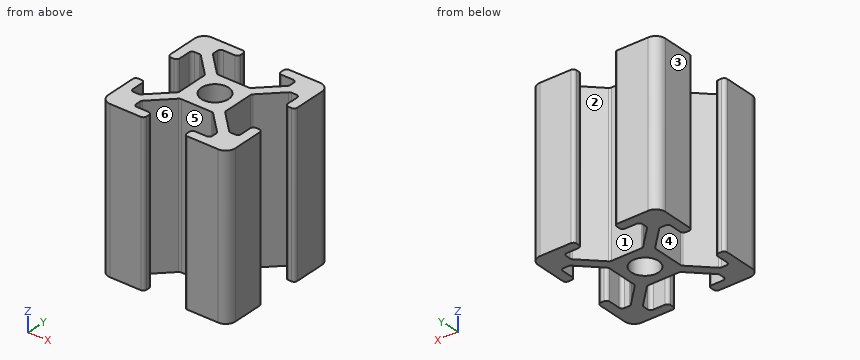
from build123d import *

# Parameters (mm, degrees)
F0_W     = 20
F0_H     = 20
F0_R     = 2.15
F2_DEPTH = 25
F3_DEPTH = 25.001
F4_R     = 1.5
F5_R     = 0.5


with BuildPart() as f2:
    # F0 (on Top) → F2 (new body)
    with BuildSketch(Plane.XY):
        Rectangle(F0_W, F0_H)
        Circle(F0_R, mode=Mode.SUBTRACT)
    extrude(amount=F2_DEPTH)

    # F1 (on face) → F3 (cut, through all)
    with BuildSketch(Plane.XY):
        Polygon((-8.5, 3.18), (-10, 3.18), (-10, -3.18), (-8.5, -3.18), (-8.5, -6), (-7.06066, -6), (-3.65, -2.58934), (-3.65, 2.58934), (-7.06066, 6), (-8.5, 6), align=None)
        Polygon((-3.18, -8.5), (-3.18, -10), (3.18, -10), (3.18, -8.5), (6, -8.5), (6, -7.06066), (2.58934, -3.65), (-2.58934, -3.65), (-6, -7.06066), (-6, -8.5), align=None)
        Polygon((10, -3.18), (10, 3.18), (8.5, 3.18), (8.5, 6), (7.06066, 6), (3.65, 2.58934), (3.65, -2.58934), (7.06066, -6), (8.5, -6), (8.5, -3.18), align=None)
        Polygon((3.18, 10), (-3.18, 10), (-3.18, 8.5), (-6, 8.5), (-6, 7.06066), (-2.58934, 3.65), (2.58934, 3.65), (6, 7.06066), (6, 8.5), (3.18, 8.5), align=None)
    extrude(amount=F3_DEPTH, mode=Mode.SUBTRACT)

    # F4
    f4_edges = [f2.edges().sort_by_distance(p)[0] for p in [
        (10, -10, 12.5),
        (-10, -10, 12.5),
        (10, 10, 12.5),
        (-10, 10, 12.5),
    ]]
    fillet(f4_edges, radius=F4_R)

    # F5
    f5_edges = [f2.edges().sort_by_distance(p)[0] for p in [
        (-3.18, -10, 12.5),
        (-10, 3.18, 12.5),
        (-3.18, 10, 12.5),
        (3.18, -10, 12.5),
        (10, 3.18, 12.5),
        (10, -3.18, 12.5),
        (-10, -3.18, 12.5),
        (3.18, 10, 12.5),
        (-6, -8.5, 12.5),
        (-3.18, -8.5, 12.5),
        (3.18, -8.5, 12.5),
        (-8.5, 3.18, 12.5),
        (-8.5, -3.18, 12.5),
        (8.5, -3.18, 12.5),
        (8.5, 3.18, 12.5),
        (3.18, 8.5, 12.5),
        (6, 8.5, 12.5),
        (8.5, 6, 12.5),
        (7.06066, 6, 12.5),
        (6, 7.06066, 12.5),
        (-2.58934, -3.65, 12.5),
        (2.58934, -3.65, 12.5),
        (3.65, 2.58934, 12.5),
        (3.65, -2.58934, 12.5),
        (-3.65, -2.58934, 12.5),
        (-3.65, 2.58934, 12.5),
        (2.58934, 3.65, 12.5),
        (-2.58934, 3.65, 12.5),
        (-6, 8.5, 12.5),
        (-6, 7.06066, 12.5),
        (-3.18, 8.5, 12.5),
        (8.5, -6, 12.5),
        (7.06066, -6, 12.5),
        (-8.5, -6, 12.5),
        (-7.06066, -6, 12.5),
        (-6, -7.06066, 12.5),
        (6, -7.06066, 12.5),
        (6, -8.5, 12.5),
        (-8.5, 6, 12.5),
        (-7.06066, 6, 12.5),
    ]]
    fillet(f5_edges, radius=F5_R)


solid = f2.part
Can you work these out from the model? Positions are in its coordinate system, mm. Face numbers are marked on the shaded views. A direction names the side the tool comes from. Give positions to 0.01 mm unless a question says otherwise; leave off trailing zeros. Order: outer loops, then holes, each group sorted by start corner. A loop starts at its lowest first (then second) coordinate and runs counter-clockwise, first axis right, second up. Notation, with made-up numbers: M 77.5,56 L 111.5,56 A19 ccw 111.5,81 Z; hole C 13.25,86.5 d10. An arc over 180 degrees is marked long. Use one line per item in the form item = value. Start each with the question number.
Item 1: For the marked faces 4, 5 and 6, which set-ups out of +Z, -Z, +X, -X, +Y, -Y let a thin tool reach every point of the face, with its end or its side?
Item 2: Will these pins go through, and if not, where does the flat tip stop? pin 1 Ø4 at (x, z) = (1, 14) entering from +Y; pin 2 Ø1.5 at (y, z) = (-2, 12) entering from -X; pin 3 Ø1 at (x, y) = (4.5, 7.5) entering from -Z; pin 4 Ø5 at (y, z) = (0.5, 17.5) entering from -X.
Item 3: We'd pull the mould along Y, two halves only. Please class the marked faces 1, 2 and 3: +Y half, -Y half, draft (parallel to the pull), parting line (faces both ways), or undercut.
Item 4: If we section it at A-A (x = 0): Write out the boundary of the cut face in (y, z), then the cut area to 3 significant figures.
Item 5: If I drill on line 1 along Y through (x, z) = (5, 4.75); line 2 along Y through (x, z) = (8, 22.5); line 3 along Y through (x, z) = (3.5, 23.5), over which ranges is the centre line in solid material (lowest first)?
Outcome:
q1.face_4 = +Z, -Z, -X
q1.face_5 = +Z, -Z, -Y
q1.face_6 = +Z, -Z
q2.pin_1 = 4.06
q2.pin_2 = -3.81
q2.pin_3 = through
q2.pin_4 = -4.06
q3.face_1 = +Y half
q3.face_2 = undercut
q3.face_3 = draft
q4.outline = M -3.65,0 L -2.15,0 L -2.15,25 L -3.65,25 Z; M 2.15,0 L 3.65,0 L 3.65,25 L 2.15,25 Z
q4.area = 75.0 mm2
q5.line_1 = -10 to -8.5, -6.06 to -3.94, 3.94 to 6.06, 8.5 to 10
q5.line_2 = -10 to -6, 6 to 10
q5.line_3 = -9.97 to -8.53, -4.56 to 4.56, 8.53 to 9.97
